Design review of the part built by this model. Coordinates are the model's own, in mm. Face numbers are marked on the shaded views. Coordinates: 2 decimals unless noted, no trailing zeros. Loops run counter-clockwise (first coordinate to the right, second up) from the corner with the lowest first, then second, coordinate; pieces in that order, holes last. Notation, with made-up numbers: M 74.25,-36.75 L 80.25,-36.75 A28 ccw 80.25,-11.75 Z; hole C 18.5,-8 d11. An arc over 180 degrees is marked long. One line per item, written item: value.
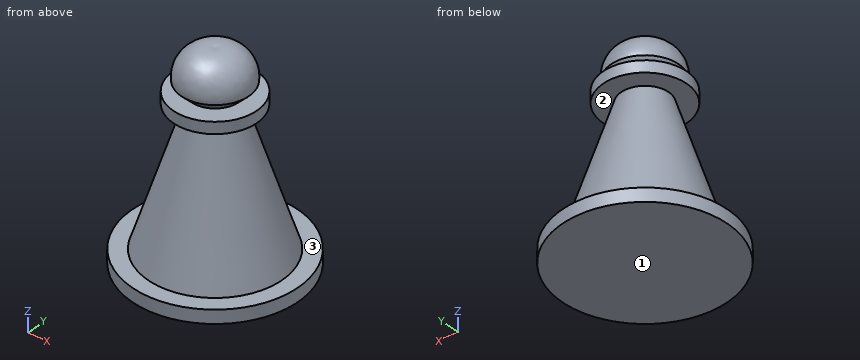
```python
from build123d import *


with BuildPart() as f1:
    # F0 (on Front) → F1 (revolve)
    with BuildSketch(Plane.XZ):
        with BuildLine():
            Line((-26.957957, 0), (0, 0))
            Line((0, 0), (0, 65.287866))
            ThreePointArc((0, 65.287866), (-8.069751, 63.231719), (-11.021761, 55.444919))
            Line((-11.021761, 55.444919), (-7.740781, 52.16394))
            Line((-7.740781, 52.16394), (-13.599676, 52.16394))
            Line((-13.599676, 52.16394), (-13.599676, 48.414249))
            Line((-13.599676, 48.414249), (-7.740781, 48.414249))
            Line((-7.740781, 48.414249), (-21.802129, 4.355352))
            Line((-21.802129, 4.355352), (-26.957957, 4.355352))
            Line((-26.957957, 4.355352), (-26.957957, 0))
        make_face()
    revolve(axis=Axis((0, 0, 32.643933), (0, 0, 1)))


solid = f1.part
```
(1) We need section C-C on x = -23. State the section outline as (y, z) points, then the cut area to 3 significant figures.
Reply:
outline: M -14.06,0 L 14.06,0 L 14.06,4.36 L -14.06,4.36 Z
area: 122 mm2
(2) We need section A-A on x = -10. State how many separate pieces and enclosed holes the cut face has, then the cut area to 3 significant figures.
Reply:
separate pieces: 3
enclosed holes: 0
area: 1,220 mm2
(3) Mouldability with a two-part tool opening along Z and no side actions: class the marked faces 1, 2 and 3 as released by +Z, released by -Z, zero draft, split by the parting line, or undercut.
Reply:
face 1: released by -Z
face 2: undercut
face 3: released by +Z
(4) We need section B-B on z = 51. State the section outline as (x, y) points.
Reply:
outline: C 0,0 d27.2
(5) Insertion check: pin 1 (12 mm diameter, centred on x = 7.5, z = 18.5, fed in from +Y); pin 2 (4 mm diameter, centred on x = 2.5, z = 54.5, fed in from +Y); pin 3 (1.5 mm diameter, centred on y = -3, z = 23, fed in from -X). Each pin has a flat end and moves straight along its axis. Give the tip position at first contact, or say it passes through.
Reply:
pin 1: stops at y = 18.41
pin 2: stops at y = 11.01
pin 3: stops at x = -15.84
(6) To check wall thickness, follow line 1 along Z through (x, y) = (20.5, -16.5); line 2 along X through (y, z) = (-18, 4); line 3 along Y through (x, z) = (-10, 22). State the ranges of each line that lie inside material, in increasing order. Write a range as [from, to].
Reply:
line 1: z = [0, 4.36]
line 2: x = [-20.07, 20.07]
line 3: y = [-12.71, 12.71]
(7) We need section D-D on z = 16. State the section outline as (x, y) points.
Reply:
outline: C 0,0 d36.17
